from build123d import *

# Parameters (mm, degrees)
BOSS_EXTRUDE2_DEPTH = 5
BOSS_EXTRUDE3_DEPTH = 20.3
BOSS_EXTRUDE4_DEPTH = 5
BOSS_EXTRUDE5_DEPTH = 50
CUT_EXTRUDE5_DEPTH  = 120.550160374
CUT_EXTRUDE6_DEPTH  = 106.793534237
BOSS_EXTRUDE6_DEPTH = 30
BOSS_EXTRUDE7_DEPTH = 20.3


with BuildPart() as part:
    # Sketch3 → Boss-Extrude2 (new body)
    with BuildSketch(Plane(origin=(0, 0, 0), x_dir=(1, 0, 0), z_dir=(0, 1, 0))):
        Polygon((-54.461524227, -2.229452052), (-41.811524227, -24.139894768), (0, -24.139894768), (0, 29.213923621), (0, 53.936652846), (-65.166780007, 16.312594867), align=None)
    boss_extrude2 = extrude(amount=BOSS_EXTRUDE2_DEPTH)

    # Sketch4 → Boss-Extrude3 (add)
    with BuildSketch(Plane(origin=(0, 5, 0), x_dir=(1, 0, 0), z_dir=(0, 1, 0))):
        Polygon((-51.961524227, -6.559579071), (0, 23.440420929), (0, 29.213923621), (0, 53.936652846), (-65.166780007, 16.312594867), (-54.461524227, -2.229452052), align=None)
    boss_extrude3 = extrude(amount=BOSS_EXTRUDE3_DEPTH)

    # Sketch5 → Boss-Extrude4 (add)
    with BuildSketch(Plane(origin=(0, 25.3, 0), x_dir=(1, 0, 0), z_dir=(0, 1, 0))):
        Polygon((-65.166780007, 16.312594867), (-41.811524227, -24.139894768), (0, -24.139894768), (0, 53.936652846), align=None)
    boss_extrude4 = extrude(amount=BOSS_EXTRUDE4_DEPTH)

    # Sketch7 → Boss-Extrude5 (add)
    with BuildSketch(Plane(origin=(0, 30.3, 0), x_dir=(1, 0, 0), z_dir=(0, 1, 0))):
        Polygon((-65.166780007, 16.312594867), (0, 53.936652846), (0, -24.139894768), (-41.811524227, -24.139894768), align=None)
    boss_extrude5 = extrude(amount=BOSS_EXTRUDE5_DEPTH)

    # Sketch12 → Cut-Extrude5 (cut, through all)
    with BuildSketch(Plane(origin=(-41.811524227, 0, 24.139894768), x_dir=(0.5000000000000006, 0, 0.8660254037844384), z_dir=(-0.8660254037844384, 0, 0.5000000000000006))):
        Polygon((-46.71051156, 80.3), (-46.71051156, 0), (-32.255495471, 0), (-10.739175318, 80.3), align=None)
    cut_extrude5 = extrude(amount=-CUT_EXTRUDE5_DEPTH, mode=Mode.SUBTRACT)

    # Sketch16 → Cut-Extrude6 (cut, through all)
    with BuildSketch(Plane(origin=(0, 0, 0), x_dir=(0, 0, -1), z_dir=(1, 0, 0))):
        Polygon((-24.139894768, 30.3), (23.326658439, 44.986202672), (12.400531522, 80.3), (-24.139894768, 80.3), align=None)
    cut_extrude6 = extrude(amount=-CUT_EXTRUDE6_DEPTH, mode=Mode.SUBTRACT)

    # Sketch17 → Boss-Extrude6 (add)
    with BuildSketch(Plane(origin=(0, 34.469205914, 10.664809425), x_dir=(1, 0, 0), z_dir=(0, 0.9553190031279326, 0.2955767282156244))):
        Polygon((-10.15, -14.10532534), (-10.15, 6.19467466), (0, 6.19467466), (0, 11.19467466), (-15.15, 11.19467466), (-15.15, -14.10532534), align=None)
    boss_extrude6 = extrude(amount=BOSS_EXTRUDE6_DEPTH)

    # Sketch18 → Boss-Extrude7 (add)
    with BuildSketch(Plane(origin=(0, 5, 0), x_dir=(1, 0, 0), z_dir=(0, 1, 0))):
        Polygon((0, -24.139894768), (-2.5, -24.139894768), (-22.477881057, 10.46281025), (0, 23.440420929), align=None)
    boss_extrude7 = extrude(amount=BOSS_EXTRUDE7_DEPTH)

    # Mirror2: Boss-Extrude2, Boss-Extrude3, Boss-Extrude4, Boss-Extrude5, Cut-Extrude5, Cut-Extrude6, Boss-Extrude6, Boss-Extrude7 across plane
    add(boss_extrude2.mirror(Plane(origin=(0, 5, -53.936652846), x_dir=(0, 0, 1), z_dir=(-1, 0, 0))))
    add(boss_extrude3.mirror(Plane(origin=(0, 5, -53.936652846), x_dir=(0, 0, 1), z_dir=(-1, 0, 0))))
    add(boss_extrude4.mirror(Plane(origin=(0, 5, -53.936652846), x_dir=(0, 0, 1), z_dir=(-1, 0, 0))))
    add(boss_extrude5.mirror(Plane(origin=(0, 5, -53.936652846), x_dir=(0, 0, 1), z_dir=(-1, 0, 0))))
    add(cut_extrude5.mirror(Plane(origin=(0, 5, -53.936652846), x_dir=(0, 0, 1), z_dir=(-1, 0, 0))), mode=Mode.SUBTRACT)
    add(cut_extrude6.mirror(Plane(origin=(0, 5, -53.936652846), x_dir=(0, 0, 1), z_dir=(-1, 0, 0))), mode=Mode.SUBTRACT)
    add(boss_extrude6.mirror(Plane(origin=(0, 5, -53.936652846), x_dir=(0, 0, 1), z_dir=(-1, 0, 0))))
    add(boss_extrude7.mirror(Plane(origin=(0, 5, -53.936652846), x_dir=(0, 0, 1), z_dir=(-1, 0, 0))))


solid = part.part
CAD build for the part. Positions are in the model's coordinates, mm. A direction names the side the tool comes from. Coordinates: 2 decimals unless noted, no trailing zeros. Order: outer loops, then holes, each group sorted by start corner. A loop starts at its lowest first (then second) coordinate and runs counter-clockwise, first axis right, second up. Notation, with made-up numbers: (37, 11) -> (85, 11) arc R9 cw to (85, 20) -> close; hole circle Ø6 at (42.5, 78.5). An arc over 180 degrees is marked (long way). Answer in a Markdown table with one row per item.
1) Band-saw the part on B-B (y = 11.5). List the corners of the cut face in (x, z), and give its area (3 significant figures).
Check values:
| item | result |
|---|---|
| outline | (-56.4, -1.13) -> (0, -33.69) -> (56.4, -1.13) -> (51.96, 6.56) -> (22.48, -10.46) -> (2.5, 24.14) -> (-2.5, 24.14) -> (-22.48, -10.46) -> (-51.96, 6.56) -> close |
| area | 2,270 mm2 |
2) Band-saw the part on C-C (x = -33.5). List the corners of the cut face in (y, z), and give its area (3 significant figures).
Check values:
| item | result |
|---|---|
| outline | (0, -17.9) -> (39.52, -5.68) -> (30.3, 24.14) -> (25.3, 24.14) -> (25.3, -4.1) -> (5, -4.1) -> (5, 24.14) -> (0, 24.14) -> close |
| area | 709 mm2 |
3) Flat gauge pins, fed straight in: P1, Ø17.5, axis at x = 25, z = 3, coming from the +Y side; P2, Ø8, axis at x = -8, y = 31.5, coming from the -Z side; P3, Ø5, axis at y = 30.5, z = -9, coming from the -X side; P4, Ø10.5, axis at x = -16.5, z = 2, coming from the -Y side. Where does each tip first touch, or does it go through?
Check values:
| item | result |
|---|---|
| P1 | y = 39.55 |
| P2 | z = -25.5 |
| P3 | x = -37.11 |
| P4 | y = 0 |
4) Which spindle directions (+Z, -Z, +X, -X, +Y, -Y) get a long thin tool onto all of the face, cutting with end or side? Do faces 1 (the face through (0.14, 50.43, 9.12)), 2 (the face through (27.07, 17.18, -16.3)), 3 (the face through (-0.212, 51.907, 4.342)). Say none if no direction does.
Check values:
| item | result |
|---|---|
| face 1 | +Z |
| face 2 | -Z, +X, +Y |
| face 3 | +X, -X, +Y |
5) Mould opens along X. For faces 4 (the face through (1, 0, 0)), 5 (the face through (15.15, 48, 16)), 6 (the face through (28, 5, 10)), 7 (the face through (-15.15, 48, 16)) say: pulls with the +X half, pulls with the -X half, needs draft (parallel to the pull), parting line crosses it, or undercut.
Check values:
| item | result |
|---|---|
| face 4 | needs draft |
| face 5 | pulls with the +X half |
| face 6 | undercut |
| face 7 | pulls with the -X half |
6) Drill centre lines: line 1 (X direction, y = 37.5, z = 18.5); line 2 (X direction, y = 15, z = -9.5); line 3 (Y direction, x = 36, z = 2.5). Where is each one in solid material? Low to high.
Check values:
| item | result |
|---|---|
| line 1 | -15.15 to -10.15, 10.15 to 15.15 |
| line 2 | -40.02 to -24.15, -21.92 to 21.92, 24.15 to 40.02 |
| line 3 | 0 to 5, 25.3 to 37 |
7) Band-saw the part on A-A (z = -5.5). List the corners of the cut face in (x, y).
Check values:
| item | result |
|---|---|
| outline | (-54.98, 0) -> (54.98, 0) -> (33.83, 39.47) -> (-33.83, 39.47) -> close; hole (-31.07, 5) -> (-19.61, 5) -> (-19.61, 25.3) -> (-31.07, 25.3) -> close; hole (19.61, 5) -> (31.07, 5) -> (31.07, 25.3) -> (19.61, 25.3) -> close |
8) Band-saw the part on D-D (z = 21.5). List the corners of the cut face in (x, y).
Check values:
| item | result |
|---|---|
| outline | (-43.34, 0) -> (43.34, 0) -> (43.34, 5) -> (4.02, 5) -> (4.02, 25.3) -> (43.34, 25.3) -> (43.34, 31.12) -> (15.15, 31.12) -> (15.15, 62.52) -> (10.15, 62.52) -> (10.15, 31.12) -> (-10.15, 31.12) -> (-10.15, 62.52) -> (-15.15, 62.52) -> (-15.15, 31.12) -> (-43.34, 31.12) -> (-43.34, 25.3) -> (-4.02, 25.3) -> (-4.02, 5) -> (-43.34, 5) -> close |
